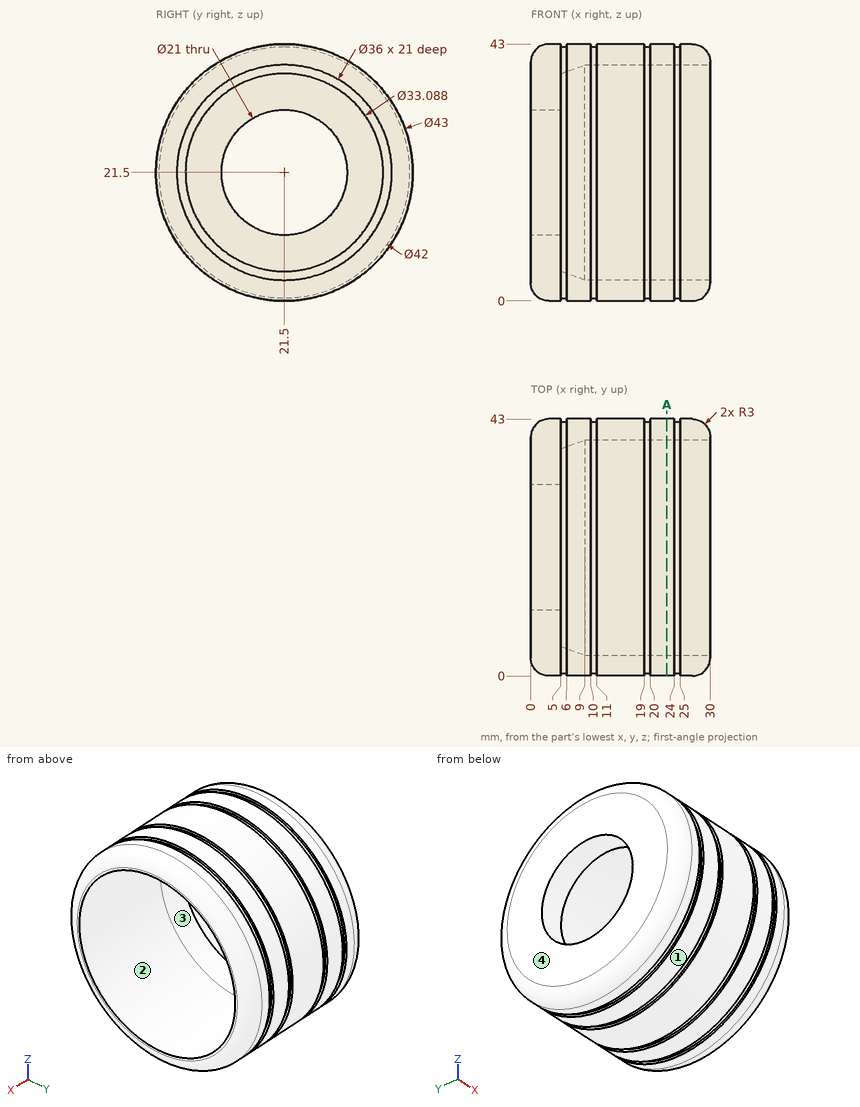
Design review of the part shown in the three views and the two pictorial views. Dimensions are in mm from the part's minimum x, y and z. Round coordinates to 2 decimals unless told otherwise and drop trailing zeros. Write each loop counter-clockwise with the first axis right and the second up, starting at its lowest first coordinate (ties: lowest second). Pieces come first, ordered by that corner, then holes.
Item 1: Consider section A-A on x = 22.75. Give the boundary of the cut face in (y, z), and give its area (3 significant figures).
Item 2: Wall thickness on L1, parallel to Y at x = 15.5, z = 21.5; L2, parallel to Y at x = 3.7, z = 21.5; L3, parallel to Z at x = 23, y = 23.5: over which ranges is each line inside the solid? List them lowest first.
Item 3: For pin 1 Ø1.5 at (x, z) = (24.5, 33) entering from -Y; pin 2 Ø13 at (y, z) = (14, 16.5) entering from -X; pin 3 Ø8 at (x, z) = (12.5, 24.5) entering from +Y; pin 4 Ø1 at (x, z) = (12.5, 26.5) entering from -Y, all flat-tipped, find the tip position at first contact; note any pin that passes through.
Item 4: Draft analysis for pull direction Y (two halves, no side actions). For the marked faces 1, 2, 3 and 4, state which applies: released by +Y, released by -Y, zero draft, split by the parting line, or undercut.
Check values:
1. outline: circle Ø43 at (21.5, 21.5); hole circle Ø36 at (21.5, 21.5)
1. area: 434 mm2
2. L1: y = 0 to 3.5, 39.5 to 43
2. L2: y = 0 to 11, 32 to 43
2. L3: z = 0.09 to 3.61, 39.39 to 42.91
3. pin 1: stops at y = 2.99
3. pin 2: stops at x = 0
3. pin 3: stops at y = 43
3. pin 4: stops at y = 0.48
4. face 1: split by the parting line
4. face 2: undercut
4. face 3: undercut
4. face 4: zero draft
